Design review of the part shown in the three views and the two pictorial views. Dimensions are in mm from the part's minimum x, y and z. Round coordinates to 2 decimals unless told otherwise and drop trailing zeros. Loops run counter-clockwise (first coordinate to the right, second up) from the corner with the lowest first, then second, coordinate; pieces in that order, holes last.
1) Insertion check: pin 1 (3 mm diameter, centred on y = 4.5, z = 98, fed in from +X). The pin has a flat end and moves straight along its axis. Give the tip position at first contact, or say it passes through.
2) Wall thickness on L1, parallel to Z at x = 277.5, y = 1.5; L2, parallel to X at y = 6, z = 117.5: over which ranges is each line inside the solid? List them lowest first.
3) Take a section at A-A (y = 4). State the section outline as (x, z) points, then the cut area to 3 significant figures.
4) Take a section at B-B (z = 133). State the section outline as (x, y) points, then the cut area to 3 significant figures.
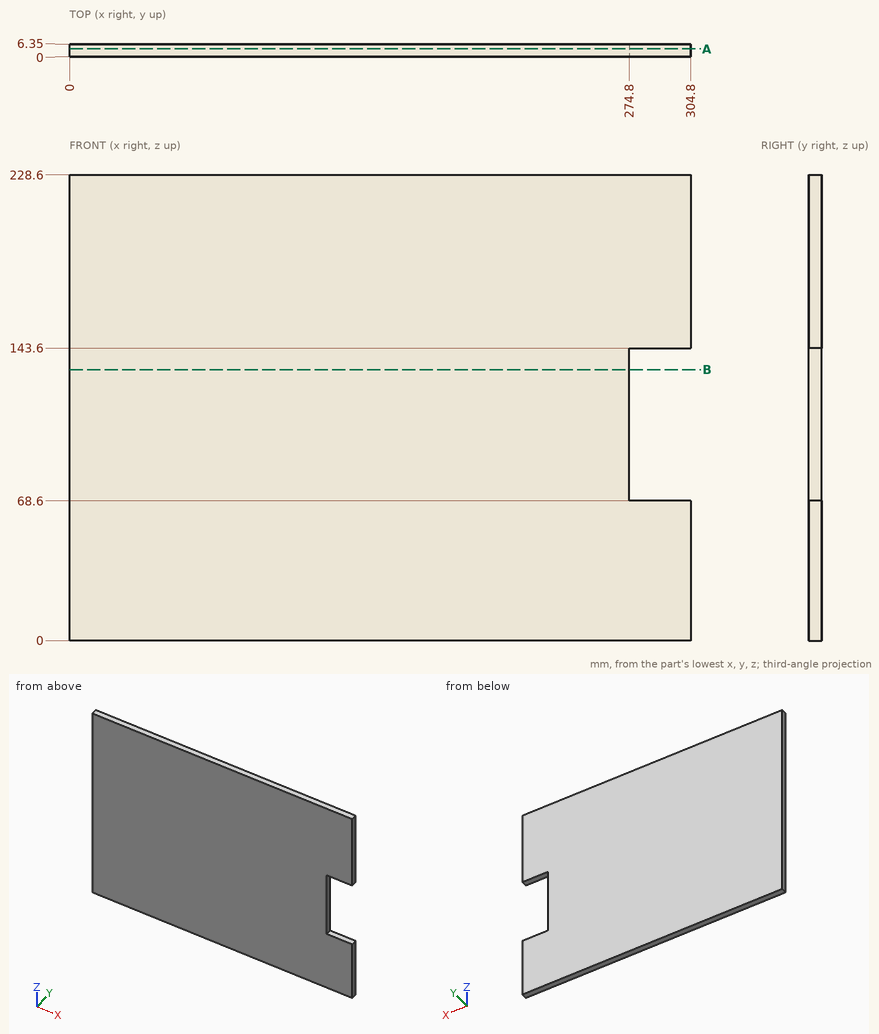
Response:
1. pin 1: stops at x = 274.8
2. L1: z = 0 to 68.6, 143.6 to 228.6
2. L2: x = 0 to 274.8
3. outline: (0, 0) - (304.8, 0) - (304.8, 68.6) - (274.8, 68.6) - (274.8, 143.6) - (304.8, 143.6) - (304.8, 228.6) - (0, 228.6) - close
3. area: 67,400 mm2
4. outline: (0, 0) - (274.8, 0) - (274.8, 6.35) - (0, 6.35) - close
4. area: 1,740 mm2
